Build history of the part. All positions in model axes, mm. Give positions to 0.01 mm unless a question says otherwise; leave off trailing zeros. Order: outer loops, then holes, each group sorted by start corner. A loop starts at its lowest first (then second) coordinate and runs counter-clockwise, first axis right, second up. Notation, with made-up numbers: (-11, 89) -> (25, 89) arc R14 ccw to (25, 112) -> close; hole circle Ø11 at (47.5, 15). An arc over 180 degrees is marked (long way). One line per question, with ' | ' between items. Start each with the question number.
(1) Cut at A-A (x = 94). Give the cut face in (y, z), then the cut area to 3 significant figures.
(2) Pin check, flat tip, straight feed: pin 1 Ø3 at (x, z) = (180, 57.62) entering from +Y. Stop position of the tip, or through.
(3) Cut at C-C (y = 2.1). Give the number of separate pieces and of enclosed holes in the cut face, then the cut area to 3 significant figures.
(4) Cut at B-B (z = 50). Give the cut face in (x, y), then the cut area to 3 significant figures.
(5) Drill centre lines: L1, parallel to Z at x = 190, y = 1.85; L2, parallel to Z at x = 180, y = 1.15; L3, parallel to X at y = 0.7, z = 43.5. Where is each one in solid material? Low to high. Write a range as from..to.
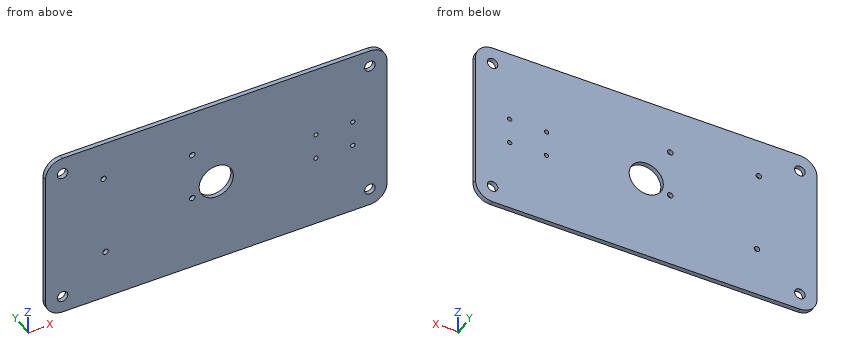
from build123d import *

# Parameters (mm, degrees)
SKETCH1_W               = 200
SKETCH1_H               = 100
BOSS_EXTRUDE1_DEPTH     = 2.6
FILLET1_R               = 10
SKETCH6_R               = 3.1
CUT_EXTRUDE6_DEPTH      = 2.6
MIRROR6_COPY_1_SKETCH_R = 3.1
MIRROR6_COPY_1_DEPTH    = 2.6
SKETCH16_R              = 1.61925
CUT_EXTRUDE9_DEPTH      = 10
SKETCH17_R              = 1.61925
CUT_EXTRUDE10_DEPTH     = 224.621913059
SKETCH18_R              = 1.61925
CUT_EXTRUDE11_DEPTH     = 224.621913059
SKETCH19_R              = 1.61925
CUT_EXTRUDE12_DEPTH     = 224.621913059
SKETCH15_R              = 10
CUT_EXTRUDE14_DEPTH     = 224.621913059
SKETCH20_R              = 1.27
CUT_EXTRUDE15_DEPTH     = 224.621913059


with BuildPart() as part:
    # Sketch1 → Boss-Extrude1 (new body)
    with BuildSketch(Plane(origin=(0, 0, 0), x_dir=(1, 0, 0), z_dir=(0, 1, 0))):
        with Locations((100, -50)):
            Rectangle(SKETCH1_W, SKETCH1_H)
    extrude(amount=BOSS_EXTRUDE1_DEPTH)

    # Fillet1
    fillet1_edges = [part.edges().sort_by_distance(p)[0] for p in [
        (0, 1.3, 0),
        (200, 1.3, 0),
        (200, 1.3, 100),
        (0, 1.3, 100),
    ]]
    fillet(fillet1_edges, radius=FILLET1_R)

    # Sketch6 → Cut-Extrude6 (cut)
    with BuildSketch(Plane.XZ):
        with Locations(Location((190, 10, 0), (0, 0, 270))):
            Circle(SKETCH6_R)
    cut_extrude6 = extrude(amount=-CUT_EXTRUDE6_DEPTH, mode=Mode.SUBTRACT)

    # Mirror5: Cut-Extrude6 across plane
    add(cut_extrude6.mirror(Plane(origin=(100, 0, 0), x_dir=(0, 0, 1), z_dir=(1, 0, 0))), mode=Mode.SUBTRACT)

    # Mirror6: Cut-Extrude6 across plane
    add(cut_extrude6.mirror(Plane.XY.offset(50)), mode=Mode.SUBTRACT)

    # Mirror6 copy 1 sketch → Mirror6 copy 1 (cut)
    with BuildSketch(Plane(origin=(200, 0, 100), x_dir=(-1, 0, 0), z_dir=(0, -1, 0))):
        with Locations(Location((190, 10, 0), (0, 0, 270))):
            Circle(MIRROR6_COPY_1_SKETCH_R)
    extrude(amount=-MIRROR6_COPY_1_DEPTH, mode=Mode.SUBTRACT)

    # Sketch16 → Cut-Extrude9 (cut)
    with BuildSketch(Plane(origin=(0, 2.6, 0), x_dir=(1, 0, 0), z_dir=(0, 1, 0))):
        with Locations(Location((35.15745, -29.37145, 0), (0, 0, 270))):
            Circle(SKETCH16_R)
    extrude(amount=-CUT_EXTRUDE9_DEPTH, mode=Mode.SUBTRACT)

    # Sketch17 → Cut-Extrude10 (cut, through all)
    with BuildSketch(Plane(origin=(0, 2.6, 0), x_dir=(1, 0, 0), z_dir=(0, 1, 0))):
        with Locations(Location((85.94475, -44.61145, 0), (0, 0, 270))):
            Circle(SKETCH17_R)
    extrude(amount=-CUT_EXTRUDE10_DEPTH, mode=Mode.SUBTRACT)

    # Sketch18 → Cut-Extrude11 (cut, through all)
    with BuildSketch(Plane(origin=(0, 2.6, 0), x_dir=(1, 0, 0), z_dir=(0, 1, 0))):
        with Locations(Location((34.01445, -77.28855, 0), (0, 0, 270))):
            Circle(SKETCH18_R)
    extrude(amount=-CUT_EXTRUDE11_DEPTH, mode=Mode.SUBTRACT)

    # Sketch19 → Cut-Extrude12 (cut, through all)
    with BuildSketch(Plane(origin=(0, 2.6, 0), x_dir=(1, 0, 0), z_dir=(0, 1, 0))):
        with Locations(Location((85.94475, -72.53875, 0), (0, 0, 270))):
            Circle(SKETCH19_R)
    extrude(amount=-CUT_EXTRUDE12_DEPTH, mode=Mode.SUBTRACT)

    # Sketch15 → Cut-Extrude14 (cut, through all)
    with BuildSketch(Plane.XZ):
        with Locations(Location((100, 50, 0), (0, 0, 270))):
            Circle(SKETCH15_R)
    extrude(amount=-CUT_EXTRUDE14_DEPTH, mode=Mode.SUBTRACT)

    # Sketch20 → Cut-Extrude15 (cut, through all)
    with BuildSketch(Plane(origin=(0, 2.6, 0), x_dir=(1, 0, 0), z_dir=(0, 1, 0))):
        with Locations(Location((158.41, -42.38, 0), (0, 0, 270))):
            Circle(SKETCH20_R)
        with Locations(Location((180, -42.38, 0), (0, 0, 270))):
            Circle(SKETCH20_R)
        with Locations(Location((158.41, -57.62, 0), (0, 0, 270))):
            Circle(SKETCH20_R)
        with Locations(Location((180, -57.62, 0), (0, 0, 270))):
            Circle(SKETCH20_R)
    extrude(amount=-CUT_EXTRUDE15_DEPTH, mode=Mode.SUBTRACT)


solid = part.part
Result set:
1) outline: (0, 0) -> (2.6, 0) -> (2.6, 42) -> (0, 42) -> close; (0, 58) -> (2.6, 58) -> (2.6, 100) -> (0, 100) -> close | area: 218 mm2
2) pin 1: stops at y = 2.6
3) separate pieces: 1 | enclosed holes: 13 | area: 19,400 mm2
4) outline: (0, 0) -> (90, 0) -> (90, 2.6) -> (0, 2.6) -> close; (110, 0) -> (200, 0) -> (200, 2.6) -> (110, 2.6) -> close | area: 468 mm2
5) L1: z = 0..6.9, 13.1..86.9, 93.1..100 | L2: z = 0..41.11, 43.65..56.35, 58.89..100 | L3: x = 0..84.77, 87.12..92.4, 107.6..157.81, 159.01..179.4, 180.6..200
